Input: part model. Units: mm. Frame: model coordinates. A direction names the side the tool comes from. Coordinates: 2 decimals unless noted, no trailing zeros. Loops run counter-clockwise (first coordinate to the right, second up) from the corner with the lowest first, then second, coordinate; pieces in that order, holes last. Notation, with made-up numbers: (42, 52) -> (80, 52) arc R13 cw to (80, 56) -> close; hole circle Ø1 at (47, 1). An arc over 180 degrees is marked (long way). Answer as a JSON object with one key per item and string values.
from build123d import *

# Parameters (mm, degrees)
ESQUISSE1_W             = 56
ESQUISSE1_H             = 40
BOSS_EXTRU_1_DEPTH      = 3
ESQUISSE2_W             = 3.8
ESQUISSE2_H             = 4
BOSS_EXTRU_2_DEPTH      = 5.8
BOSS_EXTRU_3_DEPTH      = 4
CONG_1_R                = 1
ESQUISSE4_R             = 1.6
ENL_V_MAT_EXTRU_1_DEPTH = 9.8
ESQUISSE5_R             = 17
ENL_V_MAT_EXTRU_2_DEPTH = 9.8


with BuildPart() as part:
    # Esquisse1 → Boss.-Extru.1 (new body)
    with BuildSketch(Plane.XY):
        Rectangle(ESQUISSE1_W, ESQUISSE1_H)
    extrude(amount=BOSS_EXTRU_1_DEPTH)

    # Esquisse2 → Boss.-Extru.2 (add)
    with BuildSketch(Plane.XY.offset(3)):
        with Locations((-26.1, 18)):
            Rectangle(ESQUISSE2_W, ESQUISSE2_H)
        with Locations((26.1, 18)):
            Rectangle(ESQUISSE2_W, ESQUISSE2_H)
    extrude(amount=BOSS_EXTRU_2_DEPTH)

    # Esquisse3 → Boss.-Extru.3 (add)
    with BuildSketch(Plane(origin=(0, 20, 0), x_dir=(1, 0, 0), z_dir=(0, 1, 0))):
        Polygon((-24.2, -3), (-22.4, -8.8), (-24.2, -8.8), align=None)
        Polygon((24.2, -3), (24.2, -8.8), (22.4, -8.8), align=None)
    extrude(amount=-BOSS_EXTRU_3_DEPTH)

    # Congé1
    cong_1_edges = [part.edges().sort_by_distance(p)[0] for p in [
        (23.3, 20, 5.9),
        (-23.3, 20, 5.9),
        (28, -20, 1.5),
        (-28, -20, 1.5),
        (-28, 20, 4.4),
        (28, 20, 4.4),
        (25.2, 20, 8.8),
        (-25.2, 20, 8.8),
        (0, 20, 3),
        (0, -20, 3),
        (28, -2, 3),
        (-28, -2, 3),
        (24.2, 18, 3),
        (22.4, 18, 8.8),
        (28, 18, 8.8),
        (-28, 18, 8.8),
        (-22.4, 18, 8.8),
        (-24.2, 18, 3),
    ]]
    fillet(cong_1_edges, radius=CONG_1_R)

    # Esquisse4 → Enlèv. mat.-Extru.1 (cut, through all)
    with BuildSketch(Plane(origin=(0, 0, 0), x_dir=(-1, 0, 0), z_dir=(0, 0, -1))):
        with Locations((-16.5, 16.5)):
            Circle(ESQUISSE4_R)
        with Locations((-16.5, -16.5)):
            Circle(ESQUISSE4_R)
        with Locations((16.5, 16.5)):
            Circle(ESQUISSE4_R)
        with Locations((16.5, -16.5)):
            Circle(ESQUISSE4_R)
    extrude(amount=-ENL_V_MAT_EXTRU_1_DEPTH, mode=Mode.SUBTRACT)

    # Esquisse5 → Enlèv. mat.-Extru.2 (cut, through all)
    with BuildSketch(Plane(origin=(0, 0, 0), x_dir=(-1, 0, 0), z_dir=(0, 0, -1))):
        Circle(ESQUISSE5_R)
    extrude(amount=-ENL_V_MAT_EXTRU_2_DEPTH, mode=Mode.SUBTRACT)


solid = part.part
1. Pin query (flat end, axial travel): P1, Ø2.5, axis at x = -16.5, y = 16.5, coming from the -Z side; P2, Ø12, axis at x = 0.5, y = 13.5, coming from the +Z side; P3, Ø4, axis at x = 24.5, z = 6.5, coming from the -Y side. Return the tip coordinate at first contact, or that it passes through.
Reply:
{"P1": "passes through", "P2": "stops at z = 3", "P3": "stops at y = 16"}
2. Mould query, pull axis Z, two halves, no side actions, for faces 4 (the face through (-25, 18, 8.8)), 5 (the face through (-9.139, 14.334, 1.479)), 6 (the face through (23.3, 17.5, 5.9)). Classes: pulls with the +Z half, pulls with the -Z half, needs draft (parallel to the pull), parting line crosses it, or undercut.
Reply:
{"face 4": "pulls with the +Z half", "face 5": "needs draft", "face 6": "undercut"}
3. Section query C-C (x = 20.5). Return loops of the section in (y, z).
Reply:
{"outline": "(-20, 0) -> (20, 0) -> (20, 2) arc R1 ccw to (19, 3) -> (-19, 3) arc R1 ccw to (-20, 2) -> close"}
4. Section query A-A (y = 8). Return loops of the section in (x, z), plus the area to 3 significant figures.
Reply:
{"outline": "(-28, 0) -> (-15, 0) -> (-15, 3) -> (-27, 3) arc R1 ccw to (-28, 2) -> close; (15, 0) -> (28, 0) -> (28, 2) arc R1 ccw to (27, 3) -> (15, 3) -> close", "area": "77.6 mm2"}
5. Line query: line 1 along Y through (x, z) = (0, 0.95); line 2 along X through (y, z) = (17, 3.75); line 3 along Z through (x, y) = (-21, 13.5). Output: solid intervals per line, ascending.
Reply:
{"line 1": "y = -20 to -17, 17 to 20", "line 2": "x = -28 to -23.81, 23.81 to 28", "line 3": "z = 0 to 3"}
6. Access query for faces 1 (the face through (-15.32, 17.58, 1.48)), 2 (the face through (-23.3, 17.5, 5.9)), 3 (the face through (-23.565, 19.699, 6.007)). Directions: +Z, -Z, +X, -X, +Y, -Y. A direction counts if a zero-diameter tool reaches every point of the face in a straight line with its end or side. Return the directions, or none.
Reply:
{"face 1": "+Z, -Z", "face 2": "+Y, -Y", "face 3": "+Y"}
7. Section query B-B (x = 0). Return loops of the section in (y, z), plus the area to 3 significant figures.
Reply:
{"outline": "(-20, 0) -> (-17, 0) -> (-17, 3) -> (-19, 3) arc R1 ccw to (-20, 2) -> close; (17, 0) -> (20, 0) -> (20, 2) arc R1 ccw to (19, 3) -> (17, 3) -> close", "area": "17.6 mm2"}
